Can you work these out from the drawing? Everything is in mm from the part's minimum corner. Round coordinates to 2 decimals unless told otherwise and drop trailing zeros. Loops run counter-clockwise (first coordinate to the right, second up) from the corner with the lowest first, then second, coordinate; pieces in that order, holes last. Notation, with made-up numbers: (-38.5, 1.25) - (-31.5, 1.25) arc R22 ccw to (-31.5, 28.25) - close; hole circle Ø5 at (1.25, -32). An arc over 180 degrees is marked (long way). Answer as a JSON object with one key per item and string values. Group by question number.
1) If I drill on line 1 along X through (y, z) = (1.1, 2.65); line 2 along X through (y, z) = (2.3, 3.45) (1 decimal), over which ranges is the centre line in solid material (lowest first)? Write a range as [from, to].
2) I want a section at B-B, the plane y = 1.55. Please give me the cut outline in (x, z).
3) I want a section at A-A, the plane z = 2.5. Please give me the cut outline in (x, y), then the cut area to 3 significant figures.
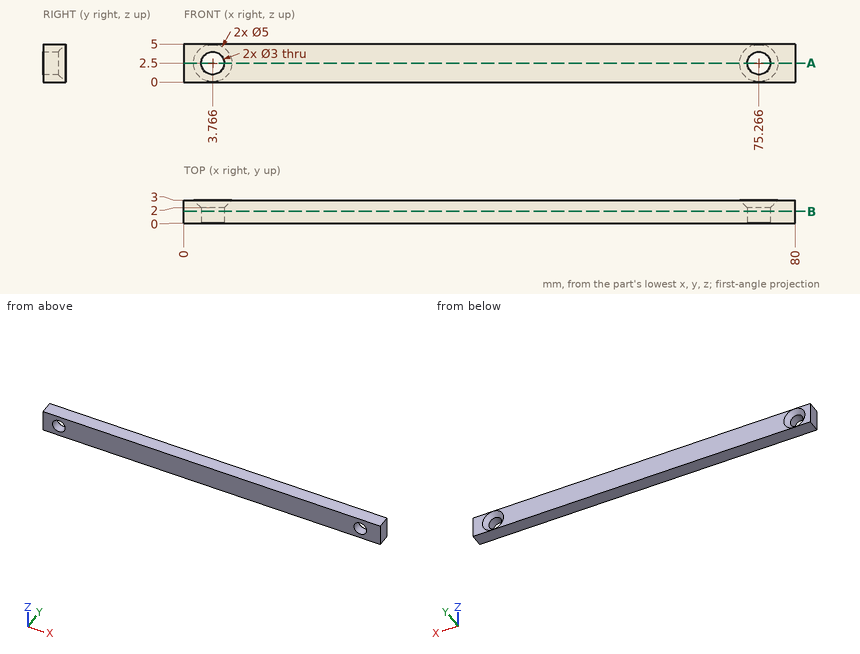
Outcome:
{
 "1": {"line 1": "[0, 2.27], [5.26, 73.77], [76.76, 80]", "line 2": "[0, 2.2], [5.3, 73.7], [76.8, 80]"},
 "2": {"outline": "(0, 0) - (80, 0) - (80, 5) - (0, 5) - close; hole circle Ø3 at (3.77, 2.5); hole circle Ø3 at (75.27, 2.5)"},
 "3": {"outline": "(0, 0) - (2.27, 0) - (2.27, 2) - (1.27, 3) - (0, 3) - close; (5.27, 0) - (73.77, 0) - (73.77, 2) - (72.77, 3) - (6.27, 3) - (5.27, 2) - close; (76.77, 0) - (80, 0) - (80, 3) - (77.77, 3) - (76.77, 2) - close", "area": "220 mm^2"}
}
